Part model, mm, in its own coordinate system. A direction names the side the tool comes from. Round coordinates to 2 decimals unless told otherwise and drop trailing zeros. Write each loop counter-clockwise with the first axis right and the second up, starting at its lowest first coordinate (ties: lowest second). Pieces come first, ordered by that corner, then holes. Notation, with made-up numbers: M 40,64.5 L 50,64.5 A35 ccw 50,98.5 Z; hole C 69,-24.75 d7. An arc over 180 degrees is marked long. Answer as a JSON object with one key per item and string values. Group by question number.
1. Two-plate mould, pull along X, no slides. Class faces 3 (the face through (17.5, 0, 24.6)), 4 (the face through (1.1, -352, 12)), 5 (the face through (25, -352, 0.898)), 6 (the face through (0, -352, 12)): +X half, -X half, draft (parallel to the pull), parting line (faces both ways), or undercut.
2. Drill centre lines: line 1 (Z direction, x = 32, y = -244.5); line 2 (X direction, y = -640, z = 0.7); line 3 (X direction, y = -641.5, z = 15.5). Where is each one in solid material? Low to high. Write a range as from..to.
3. Which spindle directions (+Z, -Z, +X, -X, +Y, -Y) get a long thin tool onto all of the face, cutting with end or side? Do faces 1 (the face through (49.1, -352, 12)), 2 (the face through (25, -352, 0)). Say none if no direction does.
4. Band-saw the part on A-A, the plane y = -384.5. Write the cut outline in (x, z).
5. Drop flat-ended pins along their axis: pin 1 (10.5 mm diameter, centred on x = 31.1, y = -21, fed in from +Z); pin 2 (6.5 mm diameter, centred on x = 31.1, y = -418, fed in from +Z). Give the stop position or say it passes through.
from build123d import *

# Parameters (mm, degrees)
F0_W     = 50
F0_H     = 25
F0_W_2   = 48
F0_H_2   = 23
F1_DEPTH = 715
F3_D     = 8
F5_R     = 6.8335490291
F6_DEPTH = 5
F7_R     = 7.0945759033
F8_DEPTH = 5


with BuildPart() as f1:
    # F0 (on Front) → F1 (new body)
    with BuildSketch(Plane.XZ):
        with Locations((25, 12.5)):
            Rectangle(F0_W, F0_H)
        with Locations((25.1003231639, 12.3982938598)):
            Rectangle(F0_W_2, F0_H_2, mode=Mode.SUBTRACT)
    extrude(amount=F1_DEPTH)

    # F3 (through all)
    with Locations(Plane(origin=(0, 0, 0), x_dir=(1, 0, 0), z_dir=(0, 0, -1))):
        with Locations((31.1003231639, 21), (31.1003231639, 205), (31.1003231639, 418), (31.1003231639, 640)):
            Hole(F3_D / 2)

    # F5 (on offset) → F6 (cut)
    with BuildSketch(Plane(origin=(0, 0, 0), x_dir=(1, 0, 0), z_dir=(0, 0, -1))):
        with Locations((22.4420260638, 0)):
            Circle(F5_R)
    extrude(amount=-F6_DEPTH, mode=Mode.SUBTRACT)

    # F7 (on offset) → F8 (cut)
    with BuildSketch(Plane(origin=(0, 0, 0), x_dir=(1, 0, 0), z_dir=(0, 0, -1))):
        with Locations((23.400099948, 715.0086760521)):
            Circle(F7_R)
    extrude(amount=-F8_DEPTH, mode=Mode.SUBTRACT)


solid = f1.part
Worked answers:
{
 "1": {"face 3": "draft", "face 4": "undercut", "face 5": "undercut", "face 6": "-X half"},
 "2": {"line 1": "z = 0..0.9, 23.9..25", "line 2": "x = 0..27.1, 35.1..50", "line 3": "x = 0..1.1, 49.1..50"},
 "3": {"face 1": "+Y, -Y", "face 2": "-Z, +X, -X, +Y, -Y"},
 "4": {"outline": "M 0,0 L 50,0 L 50,25 L 0,25 Z; hole M 1.1,0.9 L 49.1,0.9 L 49.1,23.9 L 1.1,23.9 Z"},
 "5": {"pin 1": "stops at z = 25", "pin 2": "passes through"}
}
